```python
from build123d import *

# Parameters (mm, degrees)
F0_R     = 8
F1_DEPTH = 12
F2_R     = 8.875
F2_R_2   = 8
F3_DEPTH = 2
F4_SIZE  = 1.75
F5_R     = 6
F5_R_2   = 5.875
F6_DEPTH = 0.5


with BuildPart() as f1:
    # F0 (on Top) → F1 (new body)
    with BuildSketch(Plane.XY):
        Circle(F0_R)
    extrude(amount=F1_DEPTH)

    # F2 (on face) → F3 (join)
    with BuildSketch(Plane.XY.offset(12)):
        Circle(F2_R)
        Circle(F2_R_2, mode=Mode.SUBTRACT)
        Circle(F2_R_2)
    extrude(amount=F3_DEPTH)

    # F4
    f4_edges = [f1.edges().sort_by_distance(p)[0] for p in [
        (-8.875, 0, 14),
    ]]
    chamfer(f4_edges, length=F4_SIZE)

    # F5 (on face) → F6 (cut)
    with BuildSketch(Plane.XY.offset(14)):
        Circle(F5_R)
        Circle(F5_R_2, mode=Mode.SUBTRACT)
    extrude(amount=-F6_DEPTH, mode=Mode.SUBTRACT)


solid = f1.part
```
Read the model definition and answer for the solid it produces. Units are mm, in the model's axes. A direction names the side the tool comes from. Round coordinates to 2 decimals unless told otherwise and drop trailing zeros. Write each loop counter-clockwise with the first axis right and the second up, starting at its lowest first coordinate (ties: lowest second). Pieces come first, ordered by that corner, then holes. Notation, with made-up numbers: (-3, -34) -> (5, -34) arc R20 ccw to (5, -22) -> close; hole circle Ø9 at (60, -3.5). An arc over 180 degrees is marked (long way). Answer in a Markdown table with one row per item. Add a question column.
1) Find section A-A, the plane x = 0. Determine the outline of the cut face in (y, z) (3 decimals).
2) Find section C-C, the plane z = 1.25. Determine the outline of the cut face in (x, y), and give its area (3 significant figures).
3) Given P1, Ø5, axis at x = 4, z = 5, coming from the +Y side; P2, Ø2, axis at x = -2.5, z = 6.5, coming from the -Y side; P3, Ø6, axis at y = -5, z = 9, coming from the +X side, each flat-ended and moving along its own axis, determine where each tip first touches the part or whether it passes through.
4) Consider line 1 (Y direction, x = -7, z = 11.25); line 2 (Z direction, x = -7, y = 3.75); line 3 (Z direction, x = 2, y = -8). Determine where each line is inside the solid, lowest interval first.
5) Which of the six approach directions +Z, -Z, +X, -X, +Y, -Y give full straight-line access (tool end or side, diameter ignored) to faces 1 (the face through (-5, 7, 12)), 2 (the face through (0, 0, 14))?
Findings below:
| question | item | result |
|---|---|---|
| 1 | outline | (-8.875, 12) -> (-8, 12) -> (-8, 0) -> (8, 0) -> (8, 12) -> (8.875, 12) -> (8.875, 12.25) -> (7.125, 14) -> (6, 14) -> (6, 13.5) -> (5.875, 13.5) -> (5.875, 14) -> (-5.875, 14) -> (-5.875, 13.5) -> (-6, 13.5) -> (-6, 14) -> (-7.125, 14) -> (-8.875, 12.25) -> close |
| 2 | outline | circle Ø16 at (0, 0) |
| 2 | area | 201 mm² |
| 3 | P1 | y = 7.86 |
| 3 | P2 | y = -7.86 |
| 3 | P3 | x = 7.75 |
| 4 | line 1 | -3.87 to 3.87 |
| 4 | line 2 | 0 to 13.18 |
| 4 | line 3 | 12 to 12.88 |
| 5 | face 1 | -Z |
| 5 | face 2 | +Z, +X, -X, +Y, -Y |
